The model under review builds one solid part; all positions refer to its coordinate system, in mm. Face numbers are marked on the shaded views. A direction names the side the tool comes from. Give positions to 0.01 mm unless a question says otherwise; leave off trailing zeros. Loops run counter-clockwise (first coordinate to the right, second up) from the corner with the lowest first, then second, coordinate; pieces in that order, holes last. Notation, with made-up numbers: M 3.25,62 L 26.25,62 A7 ccw 26.25,67 Z; hole C 49,42 d8. An arc over 180 degrees is marked long. Write item = value, one per line. Start each with the question number.
1. For pin 1 (2 mm diameter, centred on x = -9.5, z = 3, fed in from +Y); pin 2 (2 mm diameter, centred on y = 48.5, z = 9.5, fed in from +X); pin 3 (1 mm diameter, centred on y = 16.5, z = -7, fed in from -X), all flat-tipped, find the tip position at first contact; note any pin that passes through.
2. Draft analysis for pull direction Z (two halves, no side actions). For the marked faces 3, 4 and 5, state which applies: pulls with the +Z half, pulls with the -Z half, needs draft (parallel to the pull), parting line crosses it, or undercut.
3. For the marked faces 1 and 2, list the 3-axis set-ups (+Z, -Z, +X, -X, +Y, -Y) from which the entire face can be reached by the end or side of a thin tool; tool diameter is ignored.
4. Wall thickness on line 1 along Z through (x, y) = (0, 27.5); line 2 along Z through (x, y) = (0, 1.5): over which ranges is each line inside the solid? List them lowest first. Write a range as from..to.
5. We need section C-C on z = 5.25. Give the boundary of the cut face in (x, y), then the cut area to 3 significant figures.
6. We need section D-D on y = 60.5. Give the boundary of the cut face in (x, z), then the cut area to 3 significant figures.
7. We need section A-A on y = 41. Give the boundary of the cut face in (x, z).
8. We need section B-B on x = 0. Give the boundary of the cut face in (y, z).
from build123d import *

# Parameters (mm, degrees)
ESQUISSE2_R                  = 13
BOSS_EXTRU_1_DEPTH           = 50
ESQUISSE3_R                  = 9
ENL_V_MAT_EXTRU_1_DEPTH      = 51
ESQUISSE4_R                  = 11
ENL_V_MAT_EXTRU_2_DEPTH      = 7
ESQUISSE6_R                  = 0.75
BOSS_EXTRU_2_DEPTH           = 50
R_P_TITION_CIRCULAIRE1_COUNT = 8
ESQUISSE7_R                  = 9
BOSS_EXTRU_3_DEPTH           = 3
ESQUISSE8_R                  = 4
BOSS_EXTRU_5_DEPTH           = 14
ENL_V_MAT_EXTRU_4_DEPTH      = 14


with BuildPart() as part:
    # Esquisse2 → Boss.-Extru.1 (new body)
    with BuildSketch(Plane(origin=(0, 0, 0), x_dir=(1, 0, 0), z_dir=(0, 1, 0))):
        Circle(ESQUISSE2_R)
    extrude(amount=BOSS_EXTRU_1_DEPTH)

    # Esquisse3 → Enlèv. mat.-Extru.1 (cut, through all)
    with BuildSketch(Plane.XZ):
        Circle(ESQUISSE3_R)
    extrude(amount=-ENL_V_MAT_EXTRU_1_DEPTH, mode=Mode.SUBTRACT)

    # Esquisse4 → Enlèv. mat.-Extru.2 (cut)
    with BuildSketch(Plane.XZ):
        Circle(ESQUISSE4_R)
    extrude(amount=-ENL_V_MAT_EXTRU_2_DEPTH, mode=Mode.SUBTRACT)

    # Esquisse6 → Boss.-Extru.2 (add)
    with BuildSketch(Plane(origin=(0, 0, 0), x_dir=(-1, 0, 0), z_dir=(0, -1, 0))):
        with Locations((-13, 0)):
            Circle(ESQUISSE6_R)
    boss_extru_2 = extrude(amount=-BOSS_EXTRU_2_DEPTH)

    # Répétition circulaire1: Boss.-Extru.2 ×8 about axis
    r_p_tition_circulaire1_axis = Axis((0, 0, 0), (0, 1, 0))
    for i in range(1, R_P_TITION_CIRCULAIRE1_COUNT):
        add(boss_extru_2.rotate(r_p_tition_circulaire1_axis, i * 360 / R_P_TITION_CIRCULAIRE1_COUNT))

    # Esquisse7 → Boss.-Extru.3 (add)
    with BuildSketch(Plane(origin=(0, 50, 0), x_dir=(1, 0, 0), z_dir=(0, 1, 0))):
        Circle(ESQUISSE7_R)
    extrude(amount=-BOSS_EXTRU_3_DEPTH)

    # Esquisse8 → Boss.-Extru.5 (add)
    with BuildSketch(Plane(origin=(0, 50, 0), x_dir=(1, 0, 0), z_dir=(0, 1, 0))):
        Circle(ESQUISSE8_R)
    extrude(amount=BOSS_EXTRU_5_DEPTH)

    # Esquisse10 → Enlèv. mat.-Extru.4 (cut)
    with BuildSketch(Plane(origin=(0, 64, 0), x_dir=(1, 0, 0), z_dir=(0, 1, 0))):
        with BuildLine():
            Line((-2.009853687, -2.227215337), (-2.009853687, 2.227215337))
            ThreePointArc((-2.009853687, 2.227215337), (0, 3), (2.009853687, 2.227215337))
            Line((2.009853687, 2.227215337), (2.009853687, -2.227215337))
            ThreePointArc((2.009853687, -2.227215337), (0, -3), (-2.009853687, -2.227215337))
        make_face()
    extrude(amount=-ENL_V_MAT_EXTRU_4_DEPTH, mode=Mode.SUBTRACT)


solid = part.part
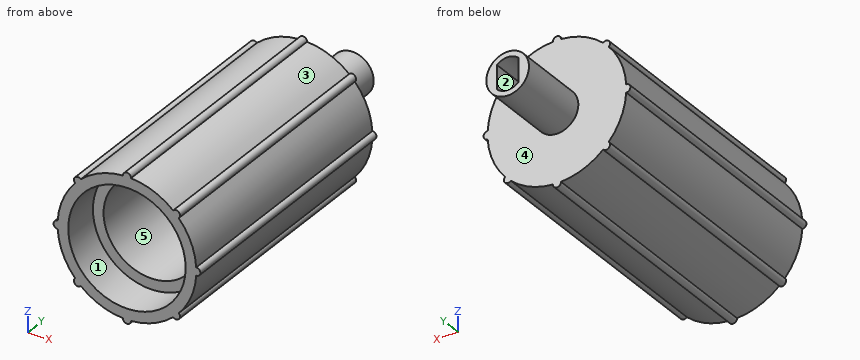
Final values:
q1.pin_1 = 50
q1.pin_2 = 9.94
q1.pin_3 = -11.26
q2.face_3 = pulls with the +Z half
q2.face_4 = needs draft
q2.face_5 = undercut
q3.face_1 = -Y
q3.face_2 = +Y
q4.line_1 = -13.75..-9, 9..13.75
q4.line_2 = -13.75..-11, 11..13.75
q5.outline = M -11.89,0 L -9.67,0 L -9.67,7 L -7.31,7 L -7.31,47 L 7.31,47 L 7.31,7 L 9.67,7 L 9.67,0 L 11.89,0 L 11.89,50 L -11.89,50 Z
q5.area = 469 mm²
q6.outline = C 0,0 d8; hole M -2.01,-2.23 A3 ccw 2.01,-2.23 L 2.01,2.23 A3 ccw -2.01,2.23 Z
q6.area = 28.1 mm²
q7.outline = M -12.98,-0.75 A13 ccw -9.71,-8.65 A0.75 ccw long -8.65,-9.71 A13 ccw -0.75,-12.98 A0.75 ccw long 0.75,-12.98 A13 ccw 8.65,-9.71 A0.75 ccw long 9.71,-8.65 A13 ccw 12.98,-0.75 A0.75 ccw long 12.98,0.75 A13 ccw 9.71,8.65 A0.75 ccw long 8.65,9.71 A13 ccw 0.75,12.98 A0.75 ccw long -0.75,12.98 A13 ccw -8.65,9.71 A0.75 ccw long -9.71,8.65 A13 ccw -12.98,0.75 A0.75 ccw long Z; hole C 0,0 d18
q8.outline = M 0,-13.75 L 50,-13.75 L 50,-4 L 64,-4 L 64,-3 L 50,-3 L 50,3 L 64,3 L 64,4 L 50,4 L 50,13.75 L 0,13.75 L 0,11 L 7,11 L 7,9 L 47,9 L 47,-9 L 7,-9 L 7,-11 L 0,-11 Z
